Input: dimensioned drawing with shaded views. Units: mm. Origin: part minimum x, y, z. A direction names the side the tool comes from. Round coordinates to 2 decimals unless told otherwise and drop trailing zeros. Loops run counter-clockwise (first coordinate to the right, second up) from the corner with the lowest first, then second, coordinate; pieces in that order, holes last. Notation, with made-up numbers: (-26.5, 57) - (-12.5, 57) arc R23 cw to (-12.5, 67) - close; hole circle Ø9 at (51.25, -2). An arc over 180 degrees is marked (long way). Answer as a JSON object with one key per item and string values. Group by question number.
Item 1: Section C-C (z = 5.75). Return the cut outline in (x, y).
Item 2: Section A-A (x = 24). Return the cut outline in (y, z), plus the area to 3 significant figures.
Item 3: Reachability of the marked faces 1 and 2 from +Z, -Z, +X, -X, +Y, -Y: full face, straight path, thin tool, end or side. Return the list, or none.
Item 4: First-contact query: pin 1 (2 mm diameter, centred on x = 24, y = 2.5, fed in from +Z); pin 2 (3 mm diameter, centred on y = 16, z = 7, fed in from -X). Flat tips, straight axial feed; report the tip coordinate or a pass-through.
Item 5: Line query: line 1 (Y direction, x = 24, z = 2); line 2 (X direction, y = 21.5, z = 6.25); line 3 (X direction, y = 10.25, z = 7). Output: solid intervals per line, ascending.
Item 6: Section D-D (y = 12). Return the cut outline in (x, z).
Item 7: Section B-B (y = 2.5). Return the cut outline in (x, z), plus the area to 3 significant figures.
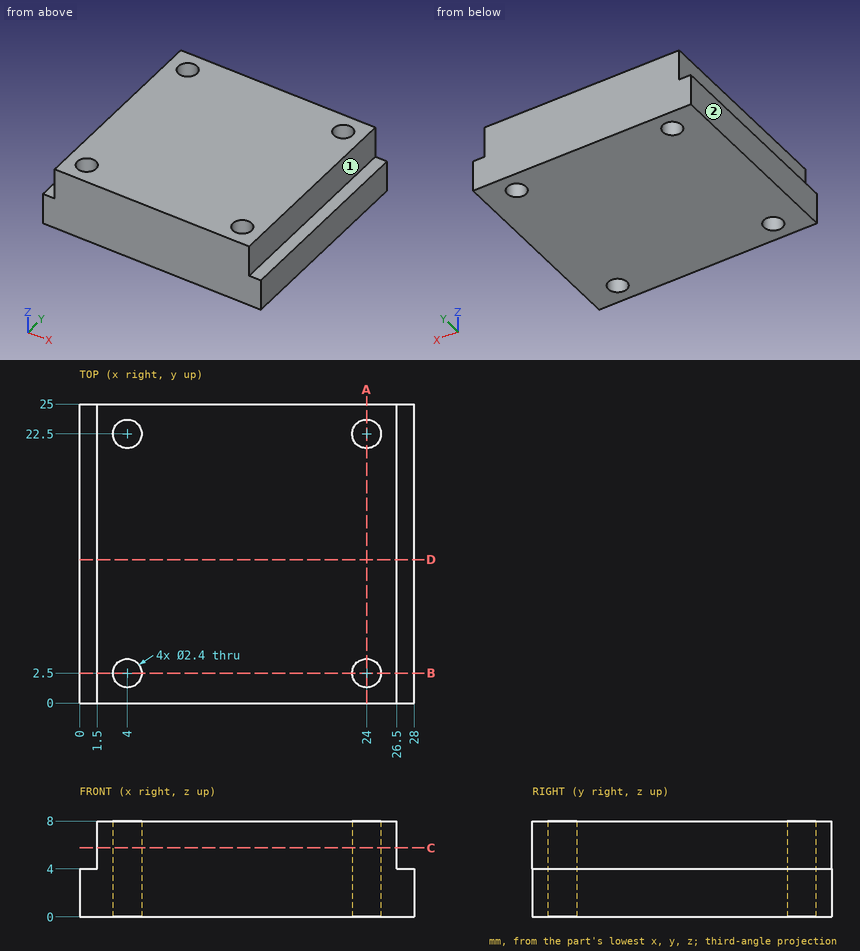
Values:
{
 "1": {"outline": "(1.5, 0) - (26.5, 0) - (26.5, 25) - (1.5, 25) - close; hole circle Ø2.4 at (4, 2.5); hole circle Ø2.4 at (4, 22.5); hole circle Ø2.4 at (24, 2.5); hole circle Ø2.4 at (24, 22.5)"},
 "2": {"outline": "(0, 0) - (1.3, 0) - (1.3, 8) - (0, 8) - close; (3.7, 0) - (21.3, 0) - (21.3, 8) - (3.7, 8) - close; (23.7, 0) - (25, 0) - (25, 8) - (23.7, 8) - close", "area": "162 mm^2"},
 "3": {"face 1": "+Z, +X, +Y, -Y", "face 2": "+Z, -Z, -X, +Y, -Y"},
 "4": {"pin 1": "passes through", "pin 2": "stops at x = 1.5"},
 "5": {"line 1": "y = 0 to 1.3, 3.7 to 21.3, 23.7 to 25", "line 2": "x = 1.5 to 3.34, 4.66 to 23.34, 24.66 to 26.5", "line 3": "x = 1.5 to 26.5"},
 "6": {"outline": "(0, 0) - (28, 0) - (28, 4) - (26.5, 4) - (26.5, 8) - (1.5, 8) - (1.5, 4) - (0, 4) - close"},
 "7": {"outline": "(0, 0) - (2.8, 0) - (2.8, 8) - (1.5, 8) - (1.5, 4) - (0, 4) - close; (5.2, 0) - (22.8, 0) - (22.8, 8) - (5.2, 8) - close; (25.2, 0) - (28, 0) - (28, 4) - (26.5, 4) - (26.5, 8) - (25.2, 8) - close", "area": "174 mm^2"}
}
